Geometry: final body of the model. Coordinates: model frame, mm. Coordinates: 2 decimals unless noted, no trailing zeros. Loops run counter-clockwise (first coordinate to the right, second up) from the corner with the lowest first, then second, coordinate; pieces in that order, holes last. Notation, with made-up numbers: M 66,76.25 L 108,76.25 A20 ccw 108,97.25 Z; hole C -5,20 d2. An arc over 180 degrees is marked long. Write item = value, one per line. Start each with the question number.
```python
from build123d import *

# Parameters (mm, degrees)
SZKIC1_W                    = 217
SZKIC1_H                    = 60
DODANIE_WYCI_GNI_CIE1_DEPTH = 3
WYTNIJ_WYCI_GNI_CIE1_DEPTH  = 226.162163784
SZKIC3_R                    = 2.1
WYTNIJ_WYCI_GNI_CIE2_DEPTH  = 226.162163784
SZKIC4_R                    = 2.1
WYTNIJ_WYCI_GNI_CIE3_DEPTH  = 226.162163784
SZKIC5_R                    = 2.1
WYTNIJ_WYCI_GNI_CIE4_DEPTH  = 226.162163784
SZKIC6_R                    = 2.1
WYTNIJ_WYCI_GNI_CIE5_DEPTH  = 226.162163784


with BuildPart() as part:
    # Szkic1 → Dodanie-wyciągnięcie1 (new body)
    with BuildSketch(Plane.XY):
        with Locations((108.5, 30)):
            Rectangle(SZKIC1_W, SZKIC1_H)
    extrude(amount=DODANIE_WYCI_GNI_CIE1_DEPTH)

    # Szkic2 → Wytnij-wyciągnięcie1 (cut, through all)
    with BuildSketch(Plane.XY.offset(3)):
        Polygon((187, 60), (217, 0), (217, 60), align=None)
    extrude(amount=-WYTNIJ_WYCI_GNI_CIE1_DEPTH, mode=Mode.SUBTRACT)

    # Szkic3 → Wytnij-wyciągnięcie2 (cut, through all)
    with BuildSketch(Plane(origin=(0, 0, 0), x_dir=(-1, 0, 0), z_dir=(0, 0, -1))):
        with Locations((-18, 24)):
            Circle(SZKIC3_R)
        with Locations((-43, 12)):
            Circle(SZKIC3_R)
        with Locations((-68, 12)):
            Circle(SZKIC3_R)
    extrude(amount=-WYTNIJ_WYCI_GNI_CIE2_DEPTH, mode=Mode.SUBTRACT)

    # Szkic4 → Wytnij-wyciągnięcie3 (cut, through all)
    with BuildSketch(Plane.XY.offset(3)):
        with Locations((93, 14.8)):
            Circle(SZKIC4_R)
        with Locations((183, 8.8)):
            Circle(SZKIC4_R)
    extrude(amount=-WYTNIJ_WYCI_GNI_CIE3_DEPTH, mode=Mode.SUBTRACT)

    # Szkic5 → Wytnij-wyciągnięcie4 (cut, through all)
    with BuildSketch(Plane.XY.offset(3)):
        with Locations((18, 46)):
            Circle(SZKIC5_R)
    extrude(amount=-WYTNIJ_WYCI_GNI_CIE4_DEPTH, mode=Mode.SUBTRACT)

    # Szkic6 → Wytnij-wyciągnięcie5 (cut, through all)
    with BuildSketch(Plane(origin=(0, 0, 0), x_dir=(-1, 0, 0), z_dir=(0, 0, -1))):
        with Locations((-52, 55)):
            Circle(SZKIC6_R)
        with Locations((-132, 55)):
            Circle(SZKIC6_R)
    extrude(amount=-WYTNIJ_WYCI_GNI_CIE5_DEPTH, mode=Mode.SUBTRACT)


solid = part.part
```
Item 1: Section query A-A (y = 55). Return the cut outline in (x, z).
Item 2: Section query B-B (x = 132). Return the cut outline in (y, z), plus the area to 3 significant figures.
Item 3: First-contact query: pin 1 (3.5 mm diameter, centred on x = 93, y = 14.8, fed in from -Z); pin 2 (6.5 mm diameter, centred on x = 18, y = 46, fed in from -Z). Flat tips, straight axial feed; report the tip coordinate or a pass-through.
Item 4: Line query: line 1 (Y direction, x = 18, z = 1.7); line 2 (X direction, y = 13, z = 2.65); line 3 (Y direction, x = 183, z = 2.15). Output: solid intervals per line, ascending. Write a range as from..to.
Item 5: Pull-direction query (X, two-part tool) for faces 1 (the flat face through (107, 30, 3)), 2 (the cylindrical face through (43.273, 14.082, 1.479)), 3 (the flat face through (202, 30, 2)); classes: released by +X, released by -X, zero draft, split by the parting line, or undercut.
Item 6: Section query C-C (z = 1.7). Count the separate pieces of the cut face and the enclosed holes in it, plus the area to 3 significant figures.
Item 7: Section query D-D (y = 29). Return the cut outline in (x, z), plus the area to 4 significant figures.
Verdict:
q1.outline = M 0,0 L 49.9,0 L 49.9,3 L 0,3 Z; M 54.1,0 L 129.9,0 L 129.9,3 L 54.1,3 Z; M 134.1,0 L 189.5,0 L 189.5,3 L 134.1,3 Z
q2.outline = M 0,0 L 52.9,0 L 52.9,3 L 0,3 Z; M 57.1,0 L 60,0 L 60,3 L 57.1,3 Z
q2.area = 167 mm2
q3.pin_1 = through
q3.pin_2 = 0
q4.line_1 = 0..21.9, 26.1..43.9, 48.1..60
q4.line_2 = 0..41.15, 44.85..66.15, 69.85..91.92, 94.08..210.5
q4.line_3 = 0..6.7, 10.9..60
q5.face_1 = zero draft
q5.face_2 = undercut
q5.face_3 = released by +X
q6.separate_pieces = 1
q6.enclosed_holes = 8
q6.area = 12,000 mm2
q7.outline = M 0,0 L 202.5,0 L 202.5,3 L 0,3 Z
q7.area = 607.5 mm2
